Check sheet for the drawn part. Datum: minimum x, y, z corner. Units: mm. Coordinates: 2 decimals unless noted, no trailing zeros. Write each loop counter-clockwise with the first axis right and the second up, starting at its lowest first coordinate (ties: lowest second). Pieces come first, ordered by that corner, then holes. Notation, with made-up numbers: (-35.75, 68.25) -> (-28.75, 68.25) arc R13 ccw to (-28.75, 90.25) -> close; hole circle Ø10 at (66.25, 66.25). An arc over 180 degrees is marked (long way). Answer in a Markdown table with one row per item.
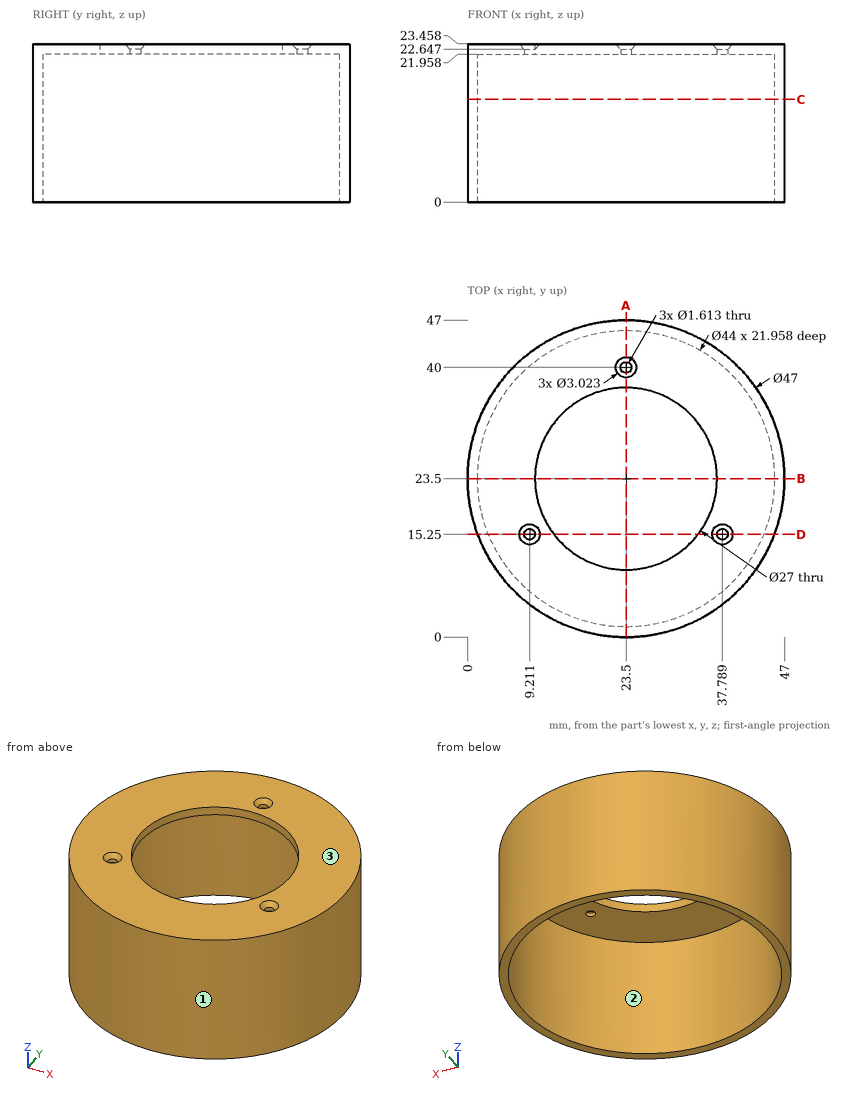
1. Sectioned sample at C-C, the plane z = 15.25. Record the cut outline in (x, y).
Findings below:
| item | result |
|---|---|
| outline | circle Ø47 at (23.5, 23.5); hole circle Ø44 at (23.5, 23.5) |
2. Go/stop test with flat-tipped pins: pin 1 (1 mm diameter, centred on x = 29.5, z = 10, fed in from -Y); pin 2 (2.5 mm diameter, centred on x = 23.5, y = 40, fed in from -Z); pin 3 (4 mm diameter, centred on x = 33, z = 4, fed in from -Y). Record where each tip stops, or that it passes through.
Findings below:
| item | result |
|---|---|
| pin 1 | stops at y = 0.65 |
| pin 2 | stops at z = 21.96 |
| pin 3 | stops at y = 1.23 |
3. Sectioned sample at A-A, the plane x = 23.5. Record the cut outline in (y, z).
Findings below:
| item | result |
|---|---|
| outline | (0, 0) -> (1.5, 0) -> (1.5, 21.96) -> (10, 21.96) -> (10, 23.46) -> (0, 23.46) -> close; (37, 21.96) -> (39.19, 21.96) -> (39.19, 22.65) -> (38.49, 23.46) -> (37, 23.46) -> close; (40.81, 21.96) -> (45.5, 21.96) -> (45.5, 0) -> (47, 0) -> (47, 23.46) -> (41.51, 23.46) -> (40.81, 22.65) -> close |
4. Release check for a two-part mould opening along X. For the marked faces 1, 2 and 3 record: released by +X, released by -X, zero draft, split by the parting line, or undercut.
Findings below:
| item | result |
|---|---|
| face 1 | split by the parting line |
| face 2 | undercut |
| face 3 | zero draft |
5. Material ranges on probe 1 along Y at (x, z) = (23.5, 22.6); probe 2 along Y at (x, z) = (23.5, 23) (1 decimal); probe 3 along Y at (x, z) = (23.5, 5.5), recorded low to high. Write a range as from..to.
Findings below:
| item | result |
|---|---|
| probe 1 | y = 0..10, 37..39.19, 40.81..47 |
| probe 2 | y = 0..10, 37..38.9, 41.1..47 |
| probe 3 | y = 0..1.5, 45.5..47 |
6. Sectioned sample at B-B, the plane y = 23.5. Record the cut outline in (x, z).
Findings below:
| item | result |
|---|---|
| outline | (0, 0) -> (1.5, 0) -> (1.5, 21.96) -> (10, 21.96) -> (10, 23.46) -> (0, 23.46) -> close; (37, 21.96) -> (45.5, 21.96) -> (45.5, 0) -> (47, 0) -> (47, 23.46) -> (37, 23.46) -> close |
7. Sectioned sample at D-D, the plane y = 15.25. Record the cut outline in (x, z) (1 decimal).
Findings below:
| item | result |
|---|---|
| outline | (1.5, 0) -> (3.1, 0) -> (3.1, 22) -> (8.4, 22) -> (8.4, 22.6) -> (7.7, 23.5) -> (1.5, 23.5) -> close; (10, 22) -> (12.8, 22) -> (12.8, 23.5) -> (10.7, 23.5) -> (10, 22.6) -> close; (34.2, 22) -> (37, 22) -> (37, 22.6) -> (36.3, 23.5) -> (34.2, 23.5) -> close; (38.6, 22) -> (43.9, 22) -> (43.9, 0) -> (45.5, 0) -> (45.5, 23.5) -> (39.3, 23.5) -> (38.6, 22.6) -> close |
